Build history of the part. All positions in model axes, mm. A direction names the side the tool comes from. Round coordinates to 2 decimals unless told otherwise and drop trailing zeros. Write each loop counter-clockwise with the first axis right and the second up, starting at its lowest first coordinate (ties: lowest second). Pieces come first, ordered by that corner, then holes. Notation, with made-up numbers: (39, 7) -> (71, 7) arc R27 cw to (71, 43) -> close; hole circle Ø10 at (-39, -11.5). An arc over 180 degrees is marked (long way). Return JSON: item names as keys, results as strings.
from build123d import *

# Parameters (mm, degrees)
F0_W     = 35
F0_H     = 30
F1_DEPTH = 1.5
F2_W     = 25
F2_H     = 3
F3_DEPTH = 1.5
F4_W     = 25
F4_H     = 1.5
F5_DEPTH = 25
F6_R     = 1.0606601718
F7_DEPTH = 1.501


# Not quite as in the source:
# - a pattern or mirror of a feature is missing from the dataset's text; its kind, count and spacing are read off the source's solid


with BuildPart() as f1:
    # F0 (on Right) → F1 (new body)
    with BuildSketch(Plane.YZ):
        Rectangle(F0_W, F0_H)
    extrude(amount=F1_DEPTH)

    # F2 (on face) → F3 (join)
    with BuildSketch(Plane.YZ.offset(1.5)):
        with Locations((0, 16.5)):
            Rectangle(F2_W, F2_H)
    f3 = extrude(amount=-F3_DEPTH)

    # F3_copies: F3 across plane
    add(f3.mirror(Plane(origin=(0, 0, 0.75), x_dir=(-1, 0, 0), z_dir=(0, 0, -1))))

    # F4 (on face) → F5 (cut)
    with BuildSketch(Plane.YZ.offset(1.5)):
        with Locations((0, -17.25)):
            Rectangle(F4_W, F4_H)
    extrude(amount=-F5_DEPTH, mode=Mode.SUBTRACT)

    # F6 (on face) → F7 (cut, through all)
    with BuildSketch(Plane.YZ.offset(1.5)):
        Polygon((-0.6338831498, 1.9119713717), (0.104722665, 1.7817352384), (0.8433284798, 1.6514991052), (2.5798102564, 11.4995766353), (1.8412044417, 11.6298127685), (1.1025986269, 11.7600489018), align=None)
        with Locations((-2.5, -12.9903810568)):
            Circle(F6_R)
        Polygon((1.9255326843, 1.3615233625), (2.6303021499, 1.105008255), (3.3350716155, 0.8484931475), (6.7552730487, 10.2454193554), (6.0505035831, 10.5019344629), (5.3457341176, 10.7584495704), align=None)
        Polygon((4.3504809472, 0.375), (5, 0), (5.6495190528, -0.375), (10.6495190528, 8.2852540378), (10, 8.6602540378), (9.3504809472, 9.0352540378), align=None)
    extrude(amount=-F7_DEPTH, mode=Mode.SUBTRACT)


solid = f1.part
Q1. Two-plate mould, pull along Y, no slides. Class faces 1 (the flat face through (0.76, 2.62, 1.11)), 2 (the flat face through (1, -12.5, -16)), 3 (the flat face through (1, 17.5, 0)), 4 (the flat face through (1.5, 0, 1)): +Y half, -Y half, draft (parallel to the pull), parting line (faces both ways), or undercut.
Verdict:
{"face 1": "undercut", "face 2": "-Y half", "face 3": "+Y half", "face 4": "draft"}
Q2. Wall check: L1, parallel to Y at x = 0.6, z = 8.5; L2, parallel to Z at x = 1, y = -2.5; L3, parallel to Y at x = 0.3, z = 7.5. Give the ranges that are in metal, low to high.
Verdict:
{"L1": "y = -17.5 to 0.53, 2.05 to 4.52, 6.12 to 9.04, 10.28 to 17.5", "L2": "z = -16.5 to -14.05, -11.93 to 18", "L3": "y = -17.5 to 0.35, 1.87 to 4.16, 5.76 to 8.46, 10.2 to 17.5"}
Q3. 3-axis set-ups, long thin cutter, end or side, ignore diameter. For faces 5 (the flat face through (0.8, 1.7, 6.5)), 6 (the flat face through (1, -15, -15)), 7 (the flat face through (1, -12.5, 16)), 8 (the flat face through (1, 12.5, 16)): which of +Z, -Z, +X, -X, +Y, -Y reach the whole face in a straight line?
Verdict:
{"face 5": "+X, -X", "face 6": "-Z, +X, -X, -Y", "face 7": "+Z, +X, -X, -Y", "face 8": "+Z, +X, -X, +Y"}
Q4. Pin check, flat tips, straight feed: pin 1 Ø0.8 at (x, y) = (1, -16) entering from -Z; pin 2 Ø3 at (y, z) = (-2.5, -12.99) entering from +X. Stop position of each tip, or through.
Verdict:
{"pin 1": "stops at z = -15", "pin 2": "stops at x = 1.5"}
Q5. Saw through at A-A on y = -2.5. List the corners of the cut face in (x, z).
Verdict:
{"outline": "(0, -16.5) -> (1.5, -16.5) -> (1.5, -14.05) -> (0, -14.05) -> close; (0, -11.93) -> (1.5, -11.93) -> (1.5, 18) -> (0, 18) -> close"}
Q6. Saw through at B-B on x = 0.4. List the corners of the cut face in (y, z) (1 decimal).
Verdict:
{"outline": "(-17.5, -15) -> (-12.5, -15) -> (-12.5, -16.5) -> (12.5, -16.5) -> (12.5, -15) -> (17.5, -15) -> (17.5, 15) -> (12.5, 15) -> (12.5, 18) -> (-12.5, 18) -> (-12.5, 15) -> (-17.5, 15) -> close; hole circle Ø2.1 at (-2.5, -13); hole (-0.6, 1.9) -> (0.8, 1.7) -> (2.6, 11.5) -> (1.1, 11.8) -> close; hole (1.9, 1.4) -> (3.3, 0.8) -> (6.8, 10.2) -> (5.3, 10.8) -> close; hole (4.4, 0.4) -> (5.6, -0.4) -> (10.6, 8.3) -> (9.4, 9) -> close"}
